For this review, use the dimensioned drawing (mm, ordinates from the lowest corner) and the shaded views. A direction names the side the tool comes from. Round coordinates to 2 decimals unless told otherwise and drop trailing zeros. Order: outer loops, then holes, each group sorted by start corner. A loop starts at its lowest first (then second) coordinate and runs counter-clockwise, first axis right, second up. Notation, with made-up numbers: (-28.5, -11.75) - (27.5, -11.75) arc R31 cw to (27.5, 12.25) - close; hole circle Ø6 at (58.5, 79.5). An arc over 180 degrees is marked (long way). Write item = value, one per line.
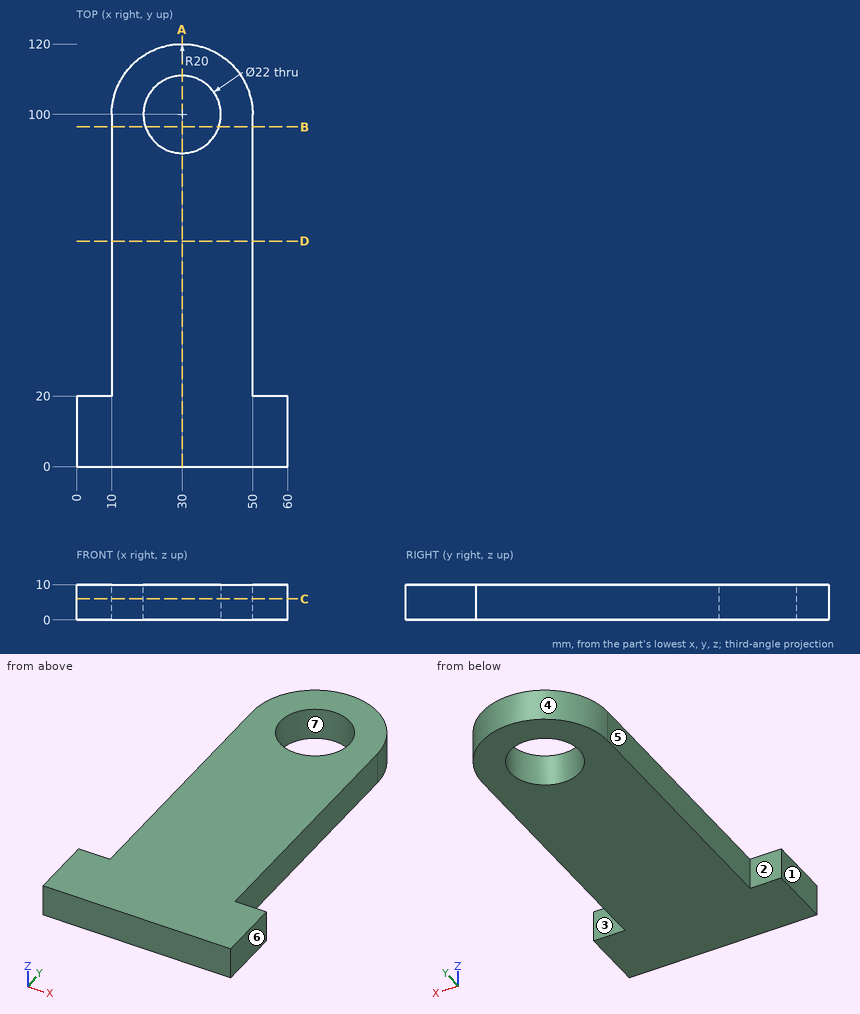
1) We need section C-C on z = 6. Write out the cut boundary in (x, y), and give its area (3 significant figures).
Findings:
outline = (0, 0) - (60, 0) - (60, 20) - (50, 20) - (50, 100) arc R20 ccw to (10, 100) - (10, 20) - (0, 20) - close; hole circle Ø22 at (30, 100)
area = 4,650 mm^2
2) The part is to be moulded in two halves that separate along X. For the marked faces 4, 5, 6 and 7, say which applies: released by +X, released by -X, zero draft, split by the parting line, or undercut.
Findings:
face_4 = split by the parting line
face_5 = released by -X
face_6 = released by +X
face_7 = undercut
3) For the marked faces 1, 2 and 3, list the 3-axis set-ups (+Z, -Z, +X, -X, +Y, -Y) from which the entire face can be reached by the end or side of a thin tool; tool diameter is ignored.
Findings:
face_1 = +Z, -Z, -X, +Y, -Y
face_2 = +Z, -Z, -X, +Y
face_3 = +Z, -Z, +X, +Y
4) We need section B-B on y = 96.5. Write out the cut boundary in (x, z), and give its area (3 significant figures).
Findings:
outline = (10, 0) - (19.57, 0) - (19.57, 10) - (10, 10) - close; (40.43, 0) - (50, 0) - (50, 10) - (40.43, 10) - close
area = 191 mm^2
5) We need section A-A on x = 30. Write out the cut boundary in (y, z), and give its area (3 significant figures).
Findings:
outline = (0, 0) - (89, 0) - (89, 10) - (0, 10) - close; (111, 0) - (120, 0) - (120, 10) - (111, 10) - close
area = 980 mm^2
6) Clearance check with flat-ended pins moving along their axes: pin 1 Ø3 at (y, z) = (36, 2) entering from -X; pin 2 Ø2 at (y, z) = (89.5, 3.5) entering from +X; pin 3 Ø2 at (x, z) = (41, 8.5) entering from +Y. State where each tip first meets the part, or that it passes through.
Findings:
pin_1 = 10
pin_2 = 50
pin_3 = 117.32
7) We need section D-D on y = 64. Write out the cut boundary in (x, z).
Findings:
outline = (10, 0) - (50, 0) - (50, 10) - (10, 10) - close
8) To check wall thickness, follow L1, parallel to Y at x = 30, z = 2; L2, parallel to Y at x = 51, z = 2; L3, parallel to Y at x = 33, z = 1.5. State the ranges of each line that lie inside material, in increasing order. Write a range as from..to.
Findings:
L1 = 0..89, 111..120
L2 = 0..20
L3 = 0..89.42, 110.58..119.77
